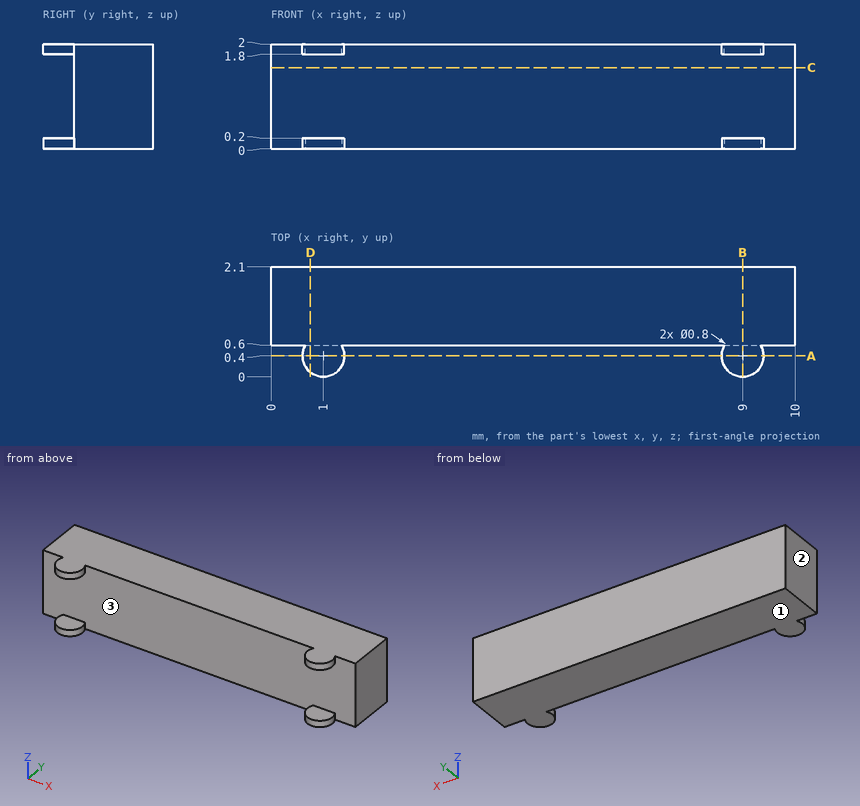
Can you work these out from the drawing? Everything is in mm from the part's minimum corner. Give positions to 0.01 mm unless a question says otherwise; leave off trailing zeros. Order: outer loops, then holes, each group sorted by start corner. A loop starts at its lowest first (then second) coordinate and runs counter-clockwise, first axis right, second up. Notation, with made-up numbers: M -19.5,23.5 L 32.5,23.5 A20 cw 32.5,43.5 Z; hole C 20,-29.75 d3. An arc over 180 degrees is marked long. Write item = value, one per line. Start each with the question number.
Q1. Suppose I cut it at D-D (x = 0.75). Write out the boundary of the cut face in (y, z), plus the area to 3 significant figures.
Q2. We'd pull the mould along X, two halves only. Please class the marked faces 1, 2 and 3: pulls with the +X half, pulls with the -X half, needs draft (parallel to the pull), parting line crosses it, or undercut.
Q3. Will this pin go through, and if not, where does the flat tip stop? pin 1 Ø1 at (x, z) = (6.5, 1) entering from -Y.
Q4. Suppose I cut it at C-C (z = 1.55). Write out the boundary of the cut face in (x, y).
Q5. Suppose I cut it at A-A (y = 0.4). Write out the boundary of the cut face in (x, z), plus the area to 3 significant figures.
Q6. I need wall thicknesses on probe 1 along Y at (x, z) = (6.75, 0.95). Which ranges of the line are inside material? Lowest first, please. Write a range as [from, to].
Q7. Suppose I cut it at B-B (x = 9). Write out the boundary of the cut face in (y, z), plus the area to 3 significant figures.
Check result:
q1.outline = M 0.09,0 L 2.1,0 L 2.1,2 L 0.09,2 L 0.09,1.8 L 0.6,1.8 L 0.6,0.2 L 0.09,0.2 Z
q1.area = 3.20 mm2
q2.face_1 = needs draft
q2.face_2 = pulls with the -X half
q2.face_3 = undercut
q3.pin_1 = 0.6
q4.outline = M 0,0.6 L 10,0.6 L 10,2.1 L 0,2.1 Z
q5.outline = M 0.6,0 L 1.4,0 L 1.4,0.2 L 0.6,0.2 Z; M 0.6,1.8 L 1.4,1.8 L 1.4,2 L 0.6,2 Z; M 8.6,0 L 9.4,0 L 9.4,0.2 L 8.6,0.2 Z; M 8.6,1.8 L 9.4,1.8 L 9.4,2 L 8.6,2 Z
q5.area = 0.640 mm2
q6.probe_1 = [0.6, 2.1]
q7.outline = M 0,0 L 2.1,0 L 2.1,2 L 0,2 L 0,1.8 L 0.6,1.8 L 0.6,0.2 L 0,0.2 Z
q7.area = 3.24 mm2
